from build123d import *

# Parameters (mm, degrees)
SKETCH1_W           = 36
SKETCH1_H           = 71.5
BOSS_EXTRUDE1_DEPTH = 8.5
SKETCH2_W           = 33
SKETCH2_H           = 62.75
CUT_EXTRUDE1_DEPTH  = 7
SKETCH4_W           = 16
SKETCH4_H           = 1.25
CUT_EXTRUDE2_DEPTH  = 6.5
FILLET1_R           = 1.25
SKETCH7_W           = 7
SKETCH7_H           = 7
BOSS_EXTRUDE4_DEPTH = 7
SKETCH8_R           = 1.55
CUT_EXTRUDE3_DEPTH  = 81.50155278
SKETCH9_R           = 3
CUT_EXTRUDE4_DEPTH  = 3.5
CUT_EXTRUDE5_DEPTH  = 80.842031537
SKETCH11_W          = 5
SKETCH11_H          = 5
BOSS_EXTRUDE8_DEPTH = 4.31
FILLET2_R           = 1.25


# Some blends are built 0.0001 mm under size
with BuildPart() as part:
    # Sketch1 → Boss-Extrude1 (new body)
    with BuildSketch(Plane(origin=(0, 0, 0), x_dir=(1, 0, 0), z_dir=(0, 1, 0))):
        with Locations((18, 35.75)):
            Rectangle(SKETCH1_W, SKETCH1_H)
    extrude(amount=BOSS_EXTRUDE1_DEPTH)

    # Sketch2 → Cut-Extrude1 (cut)
    with BuildSketch(Plane.XZ):
        with Locations((18, -32.875)):
            Rectangle(SKETCH2_W, SKETCH2_H)
    extrude(amount=-CUT_EXTRUDE1_DEPTH, mode=Mode.SUBTRACT)

    # Sketch4 → Cut-Extrude2 (cut)
    with BuildSketch(Plane(origin=(0, 0, -71.5), x_dir=(-1, 0, 0), z_dir=(0, 0, -1))):
        with Locations((-18, 0.625)):
            Rectangle(SKETCH4_W, SKETCH4_H)
    extrude(amount=-CUT_EXTRUDE2_DEPTH, mode=Mode.SUBTRACT)

    # Fillet1
    fillet1_edges = [part.edges().sort_by_distance(p)[0] for p in [
        (26, 1.25, -68.25),
        (10, 1.25, -68.25),
    ]]
    fillet(fillet1_edges, radius=FILLET1_R - 0.0001)  # a hair under: the kernel refuses the full size

    # Sketch7 → Boss-Extrude4 (add)
    with BuildSketch(Plane.XZ.offset(-7)):
        with Locations((31, -5)):
            Rectangle(SKETCH7_W, SKETCH7_H)
        with Locations((5, -5)):
            Rectangle(SKETCH7_W, SKETCH7_H)
    extrude(amount=BOSS_EXTRUDE4_DEPTH)

    # Sketch8 → Cut-Extrude3 (cut, through all)
    with BuildSketch(Plane(origin=(0, 0, 0), x_dir=(-1, 0, 0), z_dir=(0, -1, 0))):
        with Locations(Location((-31.05, 4.32, 0), (0, 0, 90))):
            Circle(SKETCH8_R)
        with Locations(Location((-32, 67.5, 0), (0, 0, 90))):
            Circle(SKETCH8_R)
        with Locations(Location((-4, 67.5, 0), (0, 0, 90))):
            Circle(SKETCH8_R)
        with Locations(Location((-4.95, 4.32, 0), (0, 0, 90))):
            Circle(SKETCH8_R)
    extrude(amount=-CUT_EXTRUDE3_DEPTH, mode=Mode.SUBTRACT)

    # Sketch9 → Cut-Extrude4 (cut)
    with BuildSketch(Plane(origin=(0, 8.5, 0), x_dir=(1, 0, 0), z_dir=(0, 1, 0))):
        with Locations(Location((4, 67.5, 0), (0, 0, 270))):
            Circle(SKETCH9_R)
        with Locations(Location((32, 67.5, 0), (0, 0, 270))):
            Circle(SKETCH9_R)
        with BuildLine():
            Line((4.95, 7.82), (0, 7.82))
            Line((0, 7.82), (0, 0))
            Line((0, 0), (8.45, 0))
            Line((8.45, 0), (8.45, 4.32))
            ThreePointArc((8.45, 4.32), (7.424873734, 6.794873734), (4.95, 7.82))
        make_face()
        with BuildLine():
            Line((27.55, 4.32), (27.55, 0))
            Line((27.55, 0), (36, 0))
            Line((36, 0), (36, 7.82))
            Line((36, 7.82), (31.05, 7.82))
            ThreePointArc((31.05, 7.82), (28.575126266, 6.794873734), (27.55, 4.32))
        make_face()
    extrude(amount=-CUT_EXTRUDE4_DEPTH, mode=Mode.SUBTRACT)

    # Sketch10 → Cut-Extrude5 (cut, through all)
    with BuildSketch(Plane.ZY.offset(-34.5)):
        with BuildLine():
            Line((-47, 5), (-43, 5))
            ThreePointArc((-43, 5), (-42, 4), (-43, 3))
            Line((-43, 3), (-47, 3))
            ThreePointArc((-47, 3), (-48, 4), (-47, 5))
        make_face()
    extrude(amount=-CUT_EXTRUDE5_DEPTH, mode=Mode.SUBTRACT)

    # Sketch11 → Boss-Extrude8 (add)
    with BuildSketch(Plane.XZ.offset(-7)):
        with Locations((4, -61.75)):
            Rectangle(SKETCH11_W, SKETCH11_H)
        with Locations((32, -61.75)):
            Rectangle(SKETCH11_W, SKETCH11_H)
    extrude(amount=BOSS_EXTRUDE8_DEPTH)

    # Fillet2
    # the kernel refuses this fillet: 1.25 mm, written as the material it takes off along each edge
    with BuildSketch(Plane(origin=(34.75, 7.25, -70.25), x_dir=(1, 0, 0), z_dir=(0, 0, -1))) as fillet2_piece_1_section:
        Polygon((0, 0), (FILLET2_R, 0), (FILLET2_R, -FILLET2_R), (0, -FILLET2_R), align=None)
    fillet2_piece_1 = extrude(amount=FILLET2_R, mode=Mode.PRIVATE)
    fillet2_piece_1 = fillet2_piece_1 - Plane(origin=(34.75, 7.25, -70.25), x_dir=(-0.7071067811865475, -0.7071067811865475, 0), z_dir=(0, 0, -1)) * Sphere(FILLET2_R, mode=Mode.PRIVATE)
    add(fillet2_piece_1, mode=Mode.SUBTRACT)
    with BuildSketch(Plane(origin=(1.25, 7.25, -70.25), x_dir=(-1, 0, 0), z_dir=(0, 0, -1))) as fillet2_piece_2_section:
        Polygon((0, 0), (FILLET2_R, 0), (FILLET2_R, FILLET2_R), (0, FILLET2_R), align=None)
    fillet2_piece_2 = extrude(amount=FILLET2_R, mode=Mode.PRIVATE)
    fillet2_piece_2 = fillet2_piece_2 - Plane(origin=(1.25, 7.25, -70.25), x_dir=(0.7071067811865475, -0.7071067811865475, 0), z_dir=(0, 0, -1)) * Sphere(FILLET2_R, mode=Mode.PRIVATE)
    add(fillet2_piece_2, mode=Mode.SUBTRACT)
    with BuildSketch(Plane(origin=(5.325, 8.5, 0), x_dir=(0, 0, -1), z_dir=(1, 0, 0))) as fillet2_piece_3:
        with BuildLine():
            CenterArc((FILLET2_R, -FILLET2_R), FILLET2_R, 90, 90)
            Line((0, -FILLET2_R), (0, 0))
            Line((0, 0), (FILLET2_R, 0))
        make_face()
    extrude(amount=25.35, mode=Mode.SUBTRACT)
    with BuildSketch(Plane(origin=(36, 8.5, -4.695), x_dir=(0, -1, 0), z_dir=(0, 0, -1))) as fillet2_piece_4:
        with BuildLine():
            CenterArc((FILLET2_R, FILLET2_R), FILLET2_R, 180, 90)
            Line((0, FILLET2_R), (0, 0))
            Line((0, 0), (FILLET2_R, 0))
        make_face()
    extrude(amount=65.555, mode=Mode.SUBTRACT)
    with BuildSketch(Plane(origin=(36, -3.125, 0), x_dir=(0, 0, -1), z_dir=(0, 1, 0))) as fillet2_piece_5:
        with BuildLine():
            CenterArc((FILLET2_R, FILLET2_R), FILLET2_R, 180, 90)
            Line((0, FILLET2_R), (0, 0))
            Line((0, 0), (FILLET2_R, 0))
        make_face()
    extrude(amount=11.25, mode=Mode.SUBTRACT)
    with BuildSketch(Plane(origin=(0, -3.125, 0), x_dir=(0, 0, -1), z_dir=(0, 1, 0))) as fillet2_piece_6:
        with BuildLine():
            CenterArc((FILLET2_R, -FILLET2_R), FILLET2_R, 90, 90)
            Line((0, -FILLET2_R), (0, 0))
            Line((0, 0), (FILLET2_R, 0))
        make_face()
    extrude(amount=11.25, mode=Mode.SUBTRACT)
    with BuildSketch(Plane(origin=(4.95, 8.5, -4.32), x_dir=(1, 0, 0), z_dir=(0, 0, 1))) as fillet2_piece_7:
        with BuildLine():
            CenterArc((3.5 + FILLET2_R, -FILLET2_R), FILLET2_R, 90, 90)
            Line((3.5, -FILLET2_R), (3.5, 0))
            Line((3.5, 0), (3.5 + FILLET2_R, 0))
        make_face()
    revolve(axis=Axis((4.95, 8.5, -4.32), (0, 1, 0)), revolution_arc=90, mode=Mode.SUBTRACT)
    with BuildSketch(Plane(origin=(4.95, 8.5, -7.82), x_dir=(0, 0, -1), z_dir=(-1, 0, 0)), Plane(origin=(39.125, 8.5, -7.82), x_dir=(0, 0, -1), z_dir=(-1, 0, 0))) as fillet2_piece_8:
        with BuildLine():
            CenterArc((FILLET2_R, FILLET2_R), FILLET2_R, 180, 90)
            Line((0, FILLET2_R), (0, 0))
            Line((0, 0), (FILLET2_R, 0))
        make_face()
    extrude(amount=8.075, mode=Mode.SUBTRACT)
    with BuildSketch(Plane(origin=(8.45, 8.5, 3.125), x_dir=(1, 0, 0), z_dir=(0, 0, -1)), Plane(origin=(27.55, 8.5, -4.32), x_dir=(-1, 0, 0), z_dir=(0, 0, 1))) as fillet2_piece_9:
        with BuildLine():
            CenterArc((FILLET2_R, FILLET2_R), FILLET2_R, 180, 90)
            Line((0, FILLET2_R), (0, 0))
            Line((0, 0), (FILLET2_R, 0))
        make_face()
    extrude(amount=7.445, mode=Mode.SUBTRACT)
    with BuildSketch(Plane(origin=(31.05, 8.5, -4.32), x_dir=(0, 0, -1), z_dir=(1, 0, 0))) as fillet2_piece_10:
        with BuildLine():
            CenterArc((3.5 + FILLET2_R, -FILLET2_R), FILLET2_R, 90, 90)
            Line((3.5, -FILLET2_R), (3.5, 0))
            Line((3.5, 0), (3.5 + FILLET2_R, 0))
        make_face()
    revolve(axis=Axis((31.05, 8.5, -4.32), (0, 1, 0)), revolution_arc=90, mode=Mode.SUBTRACT)
    with BuildSketch(Plane(origin=(34.75, 8.5, -71.5), x_dir=(0, -1, 0), z_dir=(-1, 0, 0))) as fillet2_piece_11:
        with BuildLine():
            CenterArc((FILLET2_R, FILLET2_R), FILLET2_R, 180, 90)
            Line((0, FILLET2_R), (0, 0))
            Line((0, 0), (FILLET2_R, 0))
        make_face()
    extrude(amount=33.5, mode=Mode.SUBTRACT)
    with BuildSketch(Plane(origin=(0, 8.5, -70.25), x_dir=(1, 0, 0), z_dir=(0, 0, 1))) as fillet2_piece_12:
        with BuildLine():
            CenterArc((FILLET2_R, -FILLET2_R), FILLET2_R, 90, 90)
            Line((0, -FILLET2_R), (0, 0))
            Line((0, 0), (FILLET2_R, 0))
        make_face()
    extrude(amount=65.555, mode=Mode.SUBTRACT)
    with BuildSketch(Plane(origin=(0, -3.125, -71.5), x_dir=(1, 0, 0), z_dir=(0, 1, 0))) as fillet2_piece_13:
        with BuildLine():
            CenterArc((FILLET2_R, -FILLET2_R), FILLET2_R, 90, 90)
            Line((0, -FILLET2_R), (0, 0))
            Line((0, 0), (FILLET2_R, 0))
        make_face()
    extrude(amount=10.375, mode=Mode.SUBTRACT)
    with BuildSketch(Plane(origin=(36, -3.125, -71.5), x_dir=(-1, 0, 0), z_dir=(0, 1, 0))) as fillet2_piece_14:
        with BuildLine():
            CenterArc((FILLET2_R, FILLET2_R), FILLET2_R, 180, 90)
            Line((0, FILLET2_R), (0, 0))
            Line((0, 0), (FILLET2_R, 0))
        make_face()
    extrude(amount=10.375, mode=Mode.SUBTRACT)


solid = part.part
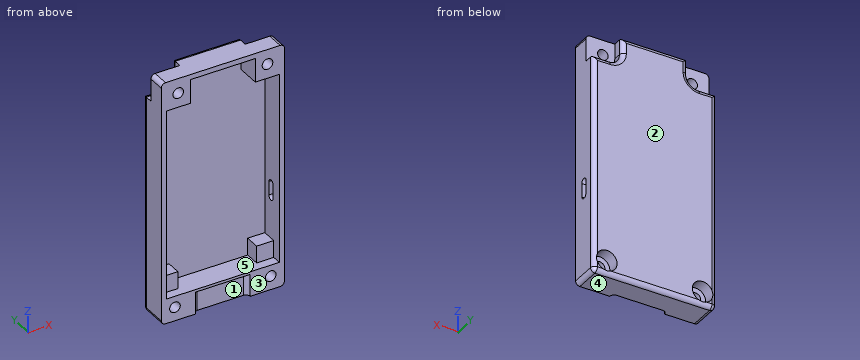
Can you work these out from the model? Positions are in its coordinate system, mm. Face numbers are marked on the shaded views. A direction names the side the tool comes from. Give positions to 0.01 mm unless a question says otherwise; leave off trailing zeros. Order: outer loops, then holes, each group sorted by start corner. A loop starts at its lowest first (then second) coordinate and runs counter-clockwise, first axis right, second up. Notation, with made-up numbers: (7.25, -14.5) - (46.25, -14.5) arc R21 ccw to (46.25, 2.5) - close; hole circle Ø9 at (-4.5, 19.5). An arc over 180 degrees is marked (long way). Write each question's results on one line, items separated by ' | '.
1) On a 3-axis mill with a long thin cutter (end or side, diameter ignored), from which of +Z, -Z, +X, -X, +Y, -Y can I reach the whole of each face in a straight line? I mean the marked faces 1 and 2. Say none if no direction works.
Final values:
face 1: -Z, -Y | face 2: +Z, -Z, +X, -X, +Y
2) Suppose I cut it at C-C, the plane y = 6.25. Write out the boundary of the cut face in (x, z), then the cut area to 3 significant figures.
Final values:
outline: (0, -70.25) arc R1.25 ccw to (1.25, -71.5) - (34.75, -71.5) arc R1.25 ccw to (36, -70.25) - (36, -7.82) - (31.05, -7.82) arc R3.5 cw to (27.55, -4.32) - (27.55, 0) - (8.45, 0) - (8.45, -4.32) arc R3.5 cw to (4.95, -7.82) - (0, -7.82) - close; hole circle Ø6 at (4, -67.5); hole (1.5, -59.25) - (6.5, -59.25) - (6.5, -64.25) - (29.5, -64.25) - (29.5, -59.25) - (34.5, -59.25) - (34.5, -8.5) - (27.5, -8.5) - (27.5, -1.5) - (8.5, -1.5) - (8.5, -8.5) - (1.5, -8.5) - close; hole circle Ø6 at (32, -67.5) | area: 467 mm^2
3) If we mould it in two halves opening along Z, with no side actions, what happens to the marked faces 3, 4 and 5? For each: pulls with the +Z half, pulls with the -Z half, needs draft (parallel to the pull), parting line crosses it, or undercut.
Final values:
face 3: needs draft | face 4: pulls with the -Z half | face 5: undercut
4) I'm going to push flat-ended pins straight in: pin 1 Ø5.5 at (x, z) = (32, -67.5) entering from +Y; pin 2 Ø1 at (x, y) = (11, 3) entering from +Z; pin 3 Ø5.5 at (x, z) = (31, -61) entering from -Y; pin 4 Ø1.1 at (x, y) = (34, 6) entering from +Z. Where does each tip first touch, or does it pass through?
Final values:
pin 1: stops at y = 5 | pin 2: stops at z = 0 | pin 3: stops at y = 2.69 | pin 4: stops at z = -7.82
5) Please list where these lines run through material, in increasing order: line 1 along X through (y, z) = (3.55, -67.5); line 2 along X through (y, z) = (6.5, -67.5); line 3 along X through (y, z) = (2.1, -4.32). Write a range as [from, to].
Final values:
line 1: x = [0, 2.45], [5.55, 30.45], [33.55, 36] | line 2: x = [0, 1], [7, 29], [35, 36] | line 3: x = [0, 3.4], [6.5, 8.5], [27.5, 29.5], [32.6, 36]
6) Suppose I cut it at A-A, the plane y = 2. Write out the boundary of the cut face in (x, z), then the cut area to 3 significant figures.
Final values:
outline: (0, -70.25) arc R1.25 ccw to (1.25, -71.5) - (34.75, -71.5) arc R1.25 ccw to (36, -70.25) - (36, -1.25) arc R1.25 ccw to (34.75, 0) - (1.25, 0) arc R1.25 ccw to (0, -1.25) - close; hole (1.5, -64.25) - (34.5, -64.25) - (34.5, -8.5) - (27.5, -8.5) - (27.5, -1.5) - (8.5, -1.5) - (8.5, -8.5) - (1.5, -8.5) - close; hole circle Ø3.1 at (4, -67.5); hole circle Ø3.1 at (4.95, -4.32); hole circle Ø3.1 at (31.05, -4.32); hole circle Ø3.1 at (32, -67.5) | area: 570 mm^2
7) Suppose I cut it at D-D, the plane z = -18.5. Write out the boundary of the cut face in (x, y), then the cut area to 3 significant figures.
Final values:
outline: (0, 0) - (1.5, 0) - (1.5, 7) - (34.5, 7) - (34.5, 0) - (36, 0) - (36, 7.25) arc R1.25 ccw to (34.75, 8.5) - (1.25, 8.5) arc R1.25 ccw to (0, 7.25) - close | area: 74.3 mm^2
8) Suppose I cut it at B-B, the plane x = 18. Write out the boundary of the cut face in (y, z), then the cut area to 3 significant figures.
Final values:
outline: (0, -65) - (1.25, -65) - (1.25, -71.5) - (7.25, -71.5) arc R1.25 ccw to (8.5, -70.25) - (8.5, -1.25) arc R1.25 ccw to (7.25, 0) - (0, 0) - (0, -1.5) - (7, -1.5) - (7, -64.25) - (0, -64.25) - close | area: 160 mm^2
